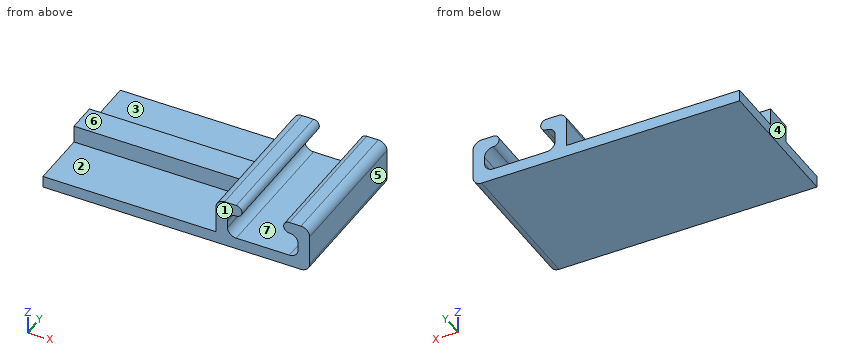
Autodesk Inventor part; units mm, degrees
ref_plane "YZ Plane" through (0, 0, 0) normal (1, 0, 0) x (0, 1, 0)
ref_plane "XZ Plane" through (0, 0, 0) normal (0, 1, 0) x (-1, 0, 0)
ref_plane "XY Plane" through (0, 0, 0) normal (0, 0, 1) x (1, 0, 0)
sketch "Hook_Base_Skt" plane through (0, 0, 0) normal (0, 1, 0) x (-1, 0, 0)
  line L0 (4.6, -2.1) -> (-4.6, -2.1)
  line L1 (-6.1, -0.6) -> (-6.1, 0.6)
  line L2 (-4.6, 2.1) -> (4.6, 2.1) construction
  line L3 (6.1, 0.6) -> (6.1, -0.6)
  line L4 (6.1, -2.1) -> (-6.1, 2.1) construction
  line L5 (-6.1, -2.1) -> (6.1, 2.1) construction
  line L6 (8.1, -4.1) -> (-6.6, -4.1)
  line L7 (-8.1, -2.6) -> (-8.1, 2.6)
  line L8 (-6.6, 4.1) -> (-4.6, 4.1)
  line L9 (8.1, 2.6) -> (8.1, -4.1)
  line L10 (8.1, -4.1) -> (-8.1, 4.1) construction
  line L11 (-8.1, -4.1) -> (8.1, 4.1) construction
  arc A0 (6.1, 0.6) -> (4.6, 2.1) centre (4.6, 0.6) ccw
  arc A1 (4.6, -2.1) -> (6.1, -0.6) centre (4.6, -0.6) ccw
  arc A2 (-6.1, -0.6) -> (-4.6, -2.1) centre (-4.6, -0.6) ccw
  arc A3 (-4.6, 2.1) -> (-6.1, 0.6) centre (-4.6, 0.6) ccw
  arc A4 (8.1, 2.6) -> (6.6, 4.1) centre (6.6, 2.6) ccw
  arc A5 (-6.6, 4.1) -> (-8.1, 2.6) centre (-6.6, 2.6) ccw
  arc A6 (-8.1, -2.6) -> (-6.6, -4.1) centre (-6.6, -2.6) ccw
  arc A7 (4.6, 4.1) -> (4.6, 2.1) centre (4.6, 3.1) ccw
  arc A8 (-4.6, 2.1) -> (-4.6, 4.1) centre (-4.6, 3.1) ccw
  line L12 (4.6, 4.1) -> (6.6, 4.1)
  line L13 (-4.6, 4.1) -> (4.6, 4.1) construction
  point P0 (0, 0)
  dimension "d29" = 12.2
  dimension "d30" = 4.2
  dimension "d31" = 2
  dimension "d32" = 2
  dimension "d34" = 1.5
extrude "Hook_Base" add sketch "Hook_Base_Skt" along normal mid plane 25
sketch "Arm_Skt" plane through (0, -12.5, 0) normal (0, -1, 0) x (1, 0, 0)
  line L0 (4.6, -2.1) -> (-4.6, -2.1)
  line L1 (0, -2.1) -> (-38, -2.1)
  line L2 (-38, -2.1) -> (-38, -4.1)
  line L3 (-38, -4.1) -> (0, -4.1)
  line L4 (6.6, -4.1) -> (-8.1, -4.1)
  line L5 (0, -4.1) -> (0, -2.1)
  point P0 (0, 0)
  dimension "d35" = 38
extrude "Arm" add sketch "Arm_Skt" against normal up to surface (25 mm away) from surface at 0
sketch "Arm_Rib_Skt" plane through (-38, -12.5, -2.1) normal (0, 0, 1) x (1, 0, 0)
  line L0 (38, 12.5) -> (0, 12.5) construction
  line L1 (0, 25) -> (0, 0) construction
  line L2 (29.9, 25) -> (29.9, 0)
  line L3 (0, 10) -> (29.9, 10)
  line L4 (29.9, 10) -> (29.9, 15)
  line L5 (29.9, 15) -> (0, 15)
  line L6 (0, 15) -> (0, 10)
  line L7 (0, 25) -> (0, 0)
  point P0 (0, 12.5)
  dimension "d38" = 5
extrude "Arm_Rib" add sketch "Arm_Rib_Skt" along normal blind 3
equation "\"d29\" = arm_width + 2 * clearance"
equation "\"d30\" = arm_thick + 2 * clearance"
equation "\"d31\" = hook_thick"
equation "\"d32\" = hook_thick"
equation "\"d34\" = general_fillet"
equation "\"d13\" = hook_width"
equation "\"d35\" = hole_to_border"
equation "\"d38\" = 0.2 * hook_width"
equation "\"d39\" = 1.5 * hook_thick"
equation "\"clearance\" = 0.1"
equation "\"arm_angle\" = 70deg"
equation "\"hole_diam\" = 3.1"
equation "\"hole_h_space\" = 126.2"
equation "\"hole_v_space\" = 65.65"
equation "\"arm_width\" = 12"
equation "\"arm_thick\" = 4"
equation "\"arm_rib_space\" = 1.25"
equation "\"arm_rib_thick\" = 2"
equation "\"base_width\" = 53"
equation "\"base_lenght\" = 138.2"
equation "\"general_fillet\" = 1.5"
equation "\"hole_to_border\" = 38"
equation "\"hook_width\" = 25"
equation "\"hook_thick\" = 2"
equation "\"rfid_width\" = 39.5"
equation "\"rfid_pin_border\" = 8"
equation "\"rfid_pin_width\" = 5"
equation "\"rfid_screw_h\" = 2.5"
equation "\"rfid_screw_v\" = 15.5"
equation "\"rfid_screw_diam\" = 3.1"
equation "\"rfid_clock_pad\" = 3"
equation "\"rfid_clock_h\" = 4.5"
equation "\"rfid_clock_v\" = 8.5"
equation "\"rfid_clock_thick\" = 1.5"
equation "\"finger_width\" = 21"
equation "\"finger_claw_h\" = 8"
equation "\"finger_claw_pad\" = 14"
equation "\"finger_claw_v\" = 7.3"
equation "\"finger_claw_clip\" = 2"
equation "\"finger_claw_ramp\" = 1"
properties part number "Sensor_Hook"
Work out the finished part from the listing and answer in its coordinate system (mm). Face numbers are marked on the shaded views. A direction names the side the tool comes from. Coordinates: 2 decimals unless noted, no trailing zeros. Loops run counter-clockwise (first coordinate to the right, second up) from the corner with the lowest first, then second, coordinate; pieces in that order, holes last. Notation, with made-up numbers: M -40,-9.75 L -15,-9.75 A16 ccw -15,6.25 Z; hole C 1,50 d9. An arc over 180 degrees is marked long. Use CSV: the item, a comma, the result in double quotes. Start each with the question number.
(1) Find section D-D, the plane z = -1.25. Give the vertices of the cut face in (x, y), then the cut area to 3 significant figures.
(2) Consider line 1 (X direction, y = -1.75, z = -0.25); line 2 (X direction, y = -6.25, z = -0.25); line 3 (Y direction, x = -33.5, z = 0). Determine where each line is inside the solid, lowest interval first.
(3) For the marked faces 1, 2 and 3, determine the directions among +Z, -Z, +X, -X, +Y, -Y from which every point of the face is accessible in a straight line to the end or side of a thin tool.
(4) Find section A-A, the plane z = 3.1. Give the vertices of the cut face in (x, y).
(5) Find section C-C, the plane x = -15.5. Give the vertices of the cut face in (y, z).
(6) Find section B-B, the plane y = -5.5. Give the vertices of the cut face in (x, z).
(7) Given pin 1 Ø4.5 at (x, y) = (-0.5, -6) entering from +Z; pin 2 Ø0.9 at (x, z) = (-19, -1) entering from +Y; pin 3 Ø1.5 at (x, y) = (-30.5, -1) entering from +Z, each flat-ended and moving along its own axis, determine where each tip first touches the part or whether it passes through.
(8) For a pull along X with two mould halves and no side action, classify the marked faces 4, 5, 6 and 7 as +X half, -X half, draft (parallel to the pull), parting line (faces both ways), or undercut.
Recorded:
1,outline,"M -38,-2.5 L -8.1,-2.5 L -8.1,-12.5 L -5.95,-12.5 L -5.95,12.5 L -8.1,12.5 L -8.1,2.5 L -38,2.5 Z; M 5.95,-12.5 L 8.1,-12.5 L 8.1,12.5 L 5.95,12.5 Z"
1,area,"257 mm^2"
2,line 1,"x = -38 to -6.1, 6.1 to 8.1"
2,line 2,"x = -8.1 to -6.1, 6.1 to 8.1"
2,line 3,"y = -2.5 to 2.5"
3,face 1,"+Z, -Z, +X, -X, -Y"
3,face 2,"+Z, -X, -Y"
3,face 3,"+Z, -X, +Y"
4,outline,"M -8.01,-12.5 L -3.6,-12.5 L -3.6,12.5 L -8.01,12.5 Z; M 3.6,-12.5 L 8.01,-12.5 L 8.01,12.5 L 3.6,12.5 Z"
5,outline,"M -12.5,-4.1 L 12.5,-4.1 L 12.5,-2.1 L 2.5,-2.1 L 2.5,0.9 L -2.5,0.9 L -2.5,-2.1 L -12.5,-2.1 Z"
6,outline,"M -38,-4.1 L 6.6,-4.1 A1.5 ccw 8.1,-2.6 L 8.1,2.6 A1.5 ccw 6.6,4.1 L 4.6,4.1 A1 ccw 4.6,2.1 A1.5 cw 6.1,0.6 L 6.1,-0.6 A1.5 cw 4.6,-2.1 L -4.6,-2.1 A1.5 cw -6.1,-0.6 L -6.1,0.6 A1.5 cw -4.6,2.1 A1 ccw -4.6,4.1 L -6.6,4.1 A1.5 ccw -8.1,2.6 L -8.1,-2.1 L -38,-2.1 Z"
7,pin 1,"stops at z = -2.1"
7,pin 2,"stops at y = 2.5"
7,pin 3,"stops at z = 0.9"
8,face 4,"-X half"
8,face 5,"+X half"
8,face 6,"draft"
8,face 7,"undercut"
